CAD build for the part. Positions are in the model's coordinates, mm. Face numbers are marked on the shaded views. A direction names the side the tool comes from. Round coordinates to 2 decimals unless told otherwise and drop trailing zeros. Write each loop counter-clockwise with the first axis right and the second up, starting at its lowest first coordinate (ties: lowest second). Pieces come first, ordered by that corner, then holes. Notation, with made-up numbers: (-8, 18) -> (35, 18) arc R12 cw to (35, 24) -> close; hole circle Ø3 at (-38, 81.5). An arc over 180 degrees is marked (long way). Put each result on its own line as item: value. Start each with the question number.
1. Saw through at C-C on z = -62.5. List the corners of the cut face in (x, y).
2. Saw through at A-A on z = -33.5. List the corners of the cut face in (x, y), and give its area (3 significant figures).
3. Drill centre lines: line 1 (X direction, y = 32.5, z = -62.5); line 2 (X direction, y = 34, z = -32.5); line 3 (X direction, y = 22.5, z = -32). Where is each one in solid material? Low to high. Write a range as from..to.
4. 3-axis set-ups, long thin cutter, end or side, ignore diameter. For the marked faces 1 and 2: which of +Z, -Z, +X, -X, +Y, -Y reach the whole face in a straight line?
5. Pull direction Y, two halves, no side cores. Call the marked faces 3, 4, 5 and 6: pulls with the +Y half, pulls with the -Y half, needs draft (parallel to the pull), parting line crosses it, or undercut.
6. Saw through at D-D on y = 22. State how many separate pieces and enclosed holes the cut face has, and give its area (3 significant figures).
7. Flat gauge pins, fed straight in: P1, Ø1.5, axis at x = 74.5, y = 11, coming from the +Z side; P2, Ø6.5, axis at x = 33.5, z = -33.5, coming from the +Y side; P3, Ø3, axis at y = 22.5, z = -21, coming from the -X side. Where does each tip first touch, or does it go through?
8. Saw through at B-B on x = 91.5. List the corners of the cut face in (y, z).
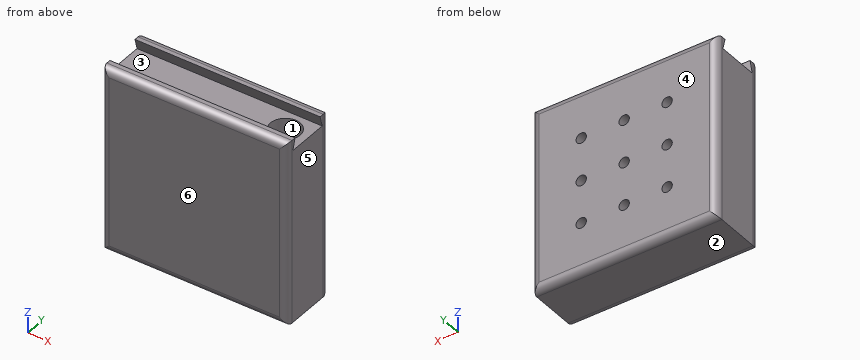
from build123d import *

# Parameters (mm, degrees)
SKETCH1_W           = 125
SKETCH1_H           = 125
BOSS_EXTRUDE1_DEPTH = 39.8
CUT_EXTRUDE1_DEPTH  = 132.8
SKETCH3_R           = 10
CUT_EXTRUDE2_DEPTH  = 40
FILLET1_R           = 5
FILLET2_R           = 5
SKETCH4_R           = 3.5
CUT_EXTRUDE3_DEPTH  = 22


with BuildPart() as part:
    # Sketch1 → Boss-Extrude1 (new body)
    with BuildSketch(Plane(origin=(0, 0, 0), x_dir=(1, 0, 0), z_dir=(0, 1, 0))):
        with Locations((62.5, 62.5)):
            Rectangle(SKETCH1_W, SKETCH1_H)
    extrude(amount=BOSS_EXTRUDE1_DEPTH)

    # Sketch2 → Cut-Extrude1 (cut)
    with BuildSketch(Plane(origin=(125, 0, 0), x_dir=(0, 0, -1), z_dir=(1, 0, 0))):
        Polygon((0, 31.9), (7.464101615, 33.9), (7.464101615, 5.9), (0, 7.9), align=None)
    extrude(amount=-CUT_EXTRUDE1_DEPTH, mode=Mode.SUBTRACT)

    # Sketch3 → Cut-Extrude2 (cut)
    with BuildSketch(Plane.XY.offset(-7.464101615)):
        with Locations((110, 19.9)):
            Circle(SKETCH3_R)
    extrude(amount=-CUT_EXTRUDE2_DEPTH, mode=Mode.SUBTRACT)

    # Fillet1
    fillet1_edges = [part.edges().sort_by_distance(p)[0] for p in [
        (125, 39.8, -62.5),
        (62.5, 39.8, -125),
        (0, 39.8, -62.5),
        (62.5, 39.8, 0),
    ]]
    fillet(fillet1_edges, radius=FILLET1_R)

    # Fillet2
    fillet2_edges = [part.edges().sort_by_distance(p)[0] for p in [
        (62.5, 0, -125),
        (125, 0, -62.5),
        (62.5, 0, 0),
        (0, 0, -62.5),
    ]]
    fillet(fillet2_edges, radius=FILLET2_R)

    # Sketch4 → Cut-Extrude3 (cut)
    with BuildSketch(Plane(origin=(0, 39.8, 0), x_dir=(1, 0, 0), z_dir=(0, 1, 0))):
        with Locations(Location((33.5, 91.5, 0), (0, 0, 270))):
            Circle(SKETCH4_R)
        with Locations(Location((62.5, 91.5, 0), (0, 0, 270))):
            Circle(SKETCH4_R)
        with Locations(Location((91.5, 91.5, 0), (0, 0, 270))):
            Circle(SKETCH4_R)
        with Locations(Location((33.5, 62.5, 0), (0, 0, 270))):
            Circle(SKETCH4_R)
        with Locations(Location((62.5, 62.5, 0), (0, 0, 270))):
            Circle(SKETCH4_R)
        with Locations(Location((91.5, 62.5, 0), (0, 0, 270))):
            Circle(SKETCH4_R)
        with Locations(Location((33.5, 33.5, 0), (0, 0, 270))):
            Circle(SKETCH4_R)
        with Locations(Location((62.5, 33.5, 0), (0, 0, 270))):
            Circle(SKETCH4_R)
        with Locations(Location((91.5, 33.5, 0), (0, 0, 270))):
            Circle(SKETCH4_R)
    extrude(amount=-CUT_EXTRUDE3_DEPTH, mode=Mode.SUBTRACT)


solid = part.part
Return value:
1. outline: (0, 5) arc R5 ccw to (5, 0) -> (120, 0) arc R5 ccw to (125, 5) -> (125, 34.8) arc R5 ccw to (120, 39.8) -> (95, 39.8) -> (95, 17.8) -> (88, 17.8) -> (88, 39.8) -> (66, 39.8) -> (66, 17.8) -> (59, 17.8) -> (59, 39.8) -> (37, 39.8) -> (37, 17.8) -> (30, 17.8) -> (30, 39.8) -> (5, 39.8) arc R5 ccw to (0, 34.8) -> close
2. outline: (0, 5) arc R5 ccw to (5, 0) -> (120, 0) arc R5 ccw to (125, 5) -> (125, 34.8) arc R5 ccw to (120, 39.8) -> (95, 39.8) -> (95, 17.8) -> (88, 17.8) -> (88, 39.8) -> (66, 39.8) -> (66, 17.8) -> (59, 17.8) -> (59, 39.8) -> (37, 39.8) -> (37, 17.8) -> (30, 17.8) -> (30, 39.8) -> (5, 39.8) arc R5 ccw to (0, 34.8) -> close; hole circle Ø20 at (110, 19.9)
2. area: 4,180 mm^2
3. line 1: x = 0..30, 37..59, 66..88, 95..125
3. line 2: x = 0..30.15, 36.85..59.15, 65.85..88.15, 94.85..125
3. line 3: x = 0..30.34, 36.66..59.34, 65.66..88.34, 94.66..100.34, 119.66..125
4. face 1: +Z
4. face 2: -Z, +X, -X, +Y, -Y
5. face 3: undercut
5. face 4: pulls with the +Y half
5. face 5: needs draft
5. face 6: pulls with the -Y half
6. separate pieces: 1
6. enclosed holes: 9
6. area: 13,600 mm^2
7. P1: stops at z = -7.46
7. P2: stops at y = 17.8
7. P3: stops at x = 0
8. outline: (0, -120) arc R5 ccw to (5, -125) -> (34.8, -125) arc R5 ccw to (39.8, -120) -> (39.8, -95) -> (17.8, -95) -> (17.8, -88) -> (39.8, -88) -> (39.8, -66) -> (17.8, -66) -> (17.8, -59) -> (39.8, -59) -> (39.8, -37) -> (17.8, -37) -> (17.8, -30) -> (39.8, -30) -> (39.8, -5) arc R5 ccw to (34.8, 0) -> (31.9, 0) -> (33.9, -7.46) -> (5.9, -7.46) -> (7.9, 0) -> (5, 0) arc R5 ccw to (0, -5) -> close
